Autodesk Inventor part; units mm, degrees
ref_plane "YZ Plane" through (0, 0, 0) normal (1, 0, 0) x (0, 1, 0)
ref_plane "XZ Plane" through (0, 0, 0) normal (0, 1, 0) x (-1, 0, 0)
ref_plane "XY Plane" through (0, 0, 0) normal (0, 0, 1) x (1, 0, 0)
sketch "Sketch1" plane through (0, 0, 0) normal (0, 0, 1) x (1, 0, 0)
  circle A0 centre (0, 0) radius 6.35 construction
  line L0 (0, 6.35) -> (-19.05, 6.35) construction
  circle A1 centre (-11.684, 0) radius 1.905 construction
  line L1 (-11.684, 0) -> (-19.05, 0) construction
  line L2 (-19.05, 0) -> (-20.3962, 0) construction
  line L3 (-20.3962, 0) -> (-20.3962, 7.4295) construction
  line L4 (-20.3962, 0) -> (-20.3962, -7.4295) construction
  line L5 (-20.3962, 7.4295) -> (-20.3962, 8.7757) construction
  circle A2 centre (-20.3962, 8.7757) radius 1.3462
  line L6 (-20.3962, -7.4295) -> (-20.3962, -8.7757) construction
  circle A3 centre (-20.3962, -8.7757) radius 1.3462
  arc A4 (-3.3157, -6.8608) -> (-4.2121, 6.35) centre (0, 0) ccw
  arc A5 (-12.6572, 2.3462) -> (-12.6572, -2.3462) centre (-11.684, 0) ccw
  line L7 (-12.6572, 2.3462) -> (-3.3157, 6.8608)
  line L8 (-12.6572, -2.3462) -> (-3.3157, -6.8608)
  line L9 (-69.6934, -33.5262) -> (46.3254, -33.5262)
  line L10 (46.3254, -33.5262) -> (46.3254, 33.5262)
  line L11 (46.3254, 33.5262) -> (-69.6934, 33.5262)
  line L12 (-69.6934, 33.5262) -> (-69.6934, -33.5262)
  dimension "d7" = 12.7
  dimension "d8" = 19.05
  dimension "d11" = 3.429
  dimension "d12" = 3.81
  dimension "d13" = 1.3462
  dimension "d14" = 7.4295
  dimension "d15" = 7.4295
  dimension "d16" = 1.3462
  dimension "d17" = 1.3462
  dimension "d18" = 15.24
  dimension "d19" = 5.08
extrude "Extrusion1" add sketch "Sketch1" along normal blind 4.572
properties part number "MOTORTOP"
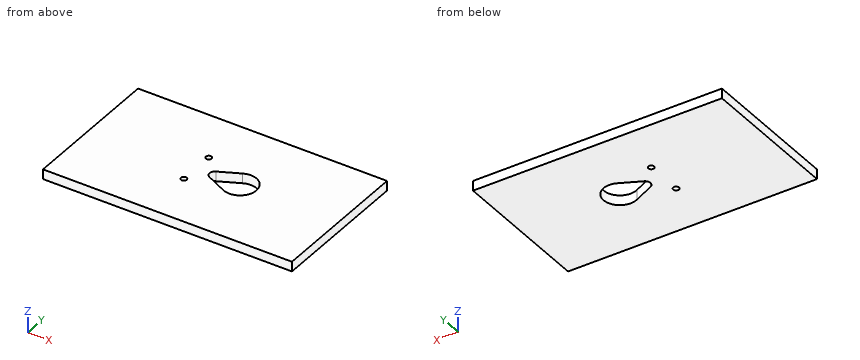
Design review of the part built by this model. Coordinates are the model's own, in mm. Coordinates: 2 decimals unless noted, no trailing zeros. Order: outer loops, then holes, each group sorted by start corner. A loop starts at its lowest first (then second) coordinate and runs counter-clockwise, first axis right, second up. Notation, with made-up numbers: (50, 71) - (99, 71) arc R36 cw to (99, 110) - close; hole circle Ø10 at (30.25, 89). An arc over 180 degrees is marked (long way). Answer in a Markdown table with one row per item.
(1) Wall thickness on line 1 along X through (y, z) = (5, 2.1); line 2 along X through (y, z) = (4.5, 2.55); line 3 along Y through (x, z) = (-4, 2.1): over which ranges is each line inside the solid? List them lowest first. Write a range as from..to.
Checked values:
| item | result |
|---|---|
| line 1 | -69.69..-7.17, 5.75..46.33 |
| line 2 | -69.69..-8.2, 6.15..46.33 |
| line 3 | -33.53..-6.53, 6.53..33.53 |
(2) Consider section A-A on x = 0. State the section outline as (y, z) points, plus the area to 3 significant figures.
Checked values:
| item | result |
|---|---|
| outline | (-33.53, 0) - (-7.62, 0) - (-7.62, 4.57) - (-33.53, 4.57) - close; (7.62, 0) - (33.53, 0) - (33.53, 4.57) - (7.62, 4.57) - close |
| area | 237 mm^2 |
(3) Consider section C-C on z = 3.75. State the section outline as (x, y) points.
Checked values:
| item | result |
|---|---|
| outline | (-69.69, -33.53) - (46.33, -33.53) - (46.33, 33.53) - (-69.69, 33.53) - close; hole circle Ø2.69 at (-20.4, -8.78); hole circle Ø2.69 at (-20.4, 8.78); hole (-12.66, -2.35) - (-3.32, -6.86) arc R7.62 ccw (long way) to (-3.32, 6.86) - (-12.66, 2.35) arc R2.54 ccw to start |
(4) Consider section B-B on x = -20.5. State the section outline as (y, z) points.
Checked values:
| item | result |
|---|---|
| outline | (-33.53, 0) - (-10.12, 0) - (-10.12, 4.57) - (-33.53, 4.57) - close; (-7.43, 0) - (7.43, 0) - (7.43, 4.57) - (-7.43, 4.57) - close; (10.12, 0) - (33.53, 0) - (33.53, 4.57) - (10.12, 4.57) - close |
(5) Clearance check with a flat-ended pin moving along its axis: pin 1 (1.6 mm diameter, centred on x = -20.4, y = -8.78, fed in from +Z). State where the tip first meets the part, or that it passes through.
Checked values:
| item | result |
|---|---|
| pin 1 | through |
